Here's how the part is built. I have some questions about the finished solid (model axes, mm). A direction names the side the tool comes from. Round coordinates to 2 decimals unless told otherwise and drop trailing zeros. Loops run counter-clockwise (first coordinate to the right, second up) from the corner with the lowest first, then second, coordinate; pieces in that order, holes last. Notation, with made-up numbers: (-40, -12) -> (-12, -12) arc R17 ccw to (-12, 16) -> close; hole circle Ø3 at (78.25, -16). An arc over 180 degrees is marked (long way). Use one line per item in the form item = value. Start each with the question number.
Item 1: If we section it at C-C (x = -29): Write out the boundary of the cut face in (y, z) (3 decimals).
Item 2: I'm going to push flat-ended pins straight in: pin 1 Ø3 at (x, y) = (18, -3.5) entering from +Z; pin 2 Ø15 at (x, z) = (-32, 43) entering from +Y (3 decimals); pin 3 Ø21 at (y, z) = (-0.5, 42.5) entering from +X (3 decimals). Where does each tip first touch, or does it pass through?
Item 3: If we section it at D-D (y = 3): Write out the boundary of the cut face in (x, z) (3 decimals), then the cut area to 3 significant figures.
Item 4: Thinking about a two-plate mould opening in X: for faces 1 (the face through (0, -11, 10)), 2 (the face through (-83, 0, 52.07)), 3 (the face through (45.921, -5, 10)), 4 (the face through (-106.479, -5, 10)), which applies, released by +X, released by -X, zero draft, split by the parting line, or undercut?
Item 5: If we section it at A-A (z = 11): Write out the boundary of the cut face in (x, y), then the cut area to 3 significant figures.
Item 6: For faces 5 (the face through (7, -21.997, 10)), 6 (the face through (-22.225, 0, 36)), 7 (the face through (-32, 9.525, 36)), which set-ups out of +Z, -Z, +X, -X, +Y, -Y let a thin tool reach every point of the face, with its end or its side?
Item 7: If we section it at B-B (z = 28.5): Write out the boundary of the cut face in (x, y) (3 decimals).
Item 8: If I drill on L1, parallel to Z at x = -32, y = 14.5; L2, parallel to X at y = -12, z = 14.5; L3, parallel to Y at x = -26, z = 32 (3 decimals), over which ranges is the centre line in solid material (lowest first)? Write a range as [from, to].
```python
from build123d import *

# Parameters (mm, degrees)
F0_R     = 12.7
F0_W     = 152.4
F0_H     = 101.6
F1_DEPTH = 20.32
F2_DEPTH = 52.07
F3_DEPTH = 52.07


with BuildPart() as f1:
    # F0 (on Top) → F1 (new body)
    with BuildSketch(Plane.XY):
        with Locations((-82.55, 0)):
            Circle(F0_R)
        with Locations((-30.279235, -4.731591)):
            Rectangle(F0_W, F0_H)
        Polygon((-6.35, -21.997045), (6.35, 0), (19.05, -21.997045), align=None, mode=Mode.SUBTRACT)
        with Locations((-82.55, 0)):
            Circle(F0_R, mode=Mode.SUBTRACT)
        Polygon((-22.225, 9.525), (-22.225, 0), (-22.225, -9.525), (-41.275, -9.525), (-41.275, 0), (-41.275, 9.525), align=None, mode=Mode.SUBTRACT)
    extrude(amount=F1_DEPTH)

    # F0 (on Top) → F2 (join)
    with BuildSketch(Plane.XY):
        Polygon((-22.225, -9.525), (-22.225, 0), (-31.75, 0), (-41.275, 0), (-41.275, -9.525), align=None)
        Polygon((-31.75, 0), (-22.225, 0), (-22.225, 9.525), (-41.275, 9.525), (-41.275, 0), align=None)
    extrude(amount=F2_DEPTH)

    # F0 (on Top) → F3 (join)
    with BuildSketch(Plane.XY):
        with Locations((-82.55, 0)):
            Circle(F0_R)
    extrude(amount=F3_DEPTH)


solid = f1.part
```
Values found:
q1.outline = (-55.532, 0) -> (46.068, 0) -> (46.068, 20.32) -> (9.525, 20.32) -> (9.525, 52.07) -> (-9.525, 52.07) -> (-9.525, 20.32) -> (-55.532, 20.32) -> close
q2.pin_1 = 20.32
q2.pin_2 = 9.525
q2.pin_3 = -22.225
q3.outline = (-106.479, 0) -> (45.921, 0) -> (45.921, 20.32) -> (-22.225, 20.32) -> (-22.225, 52.07) -> (-41.275, 52.07) -> (-41.275, 20.32) -> (-70.209, 20.32) -> (-70.209, 52.07) -> (-94.891, 52.07) -> (-94.891, 20.32) -> (-106.479, 20.32) -> close
q3.area = 4,490 mm2
q4.face_1 = undercut
q4.face_2 = zero draft
q4.face_3 = released by +X
q4.face_4 = released by -X
q5.outline = (-106.48, -55.53) -> (45.92, -55.53) -> (45.92, 46.07) -> (-106.48, 46.07) -> close; hole (-6.35, -22) -> (19.05, -22) -> (6.35, 0) -> close
q5.area = 15,200 mm2
q6.face_5 = +Z, -Z
q6.face_6 = +Z, +X, +Y, -Y
q6.face_7 = +Z, +X, +Y
q7.outline = circle Ø25.4 at (-82.55, 0); (-41.275, -9.525) -> (-22.225, -9.525) -> (-22.225, 9.525) -> (-41.275, 9.525) -> close
q8.L1 = [0, 20.32]
q8.L2 = [-106.48, -0.58], [13.28, 45.92]
q8.L3 = [-9.525, 9.525]
